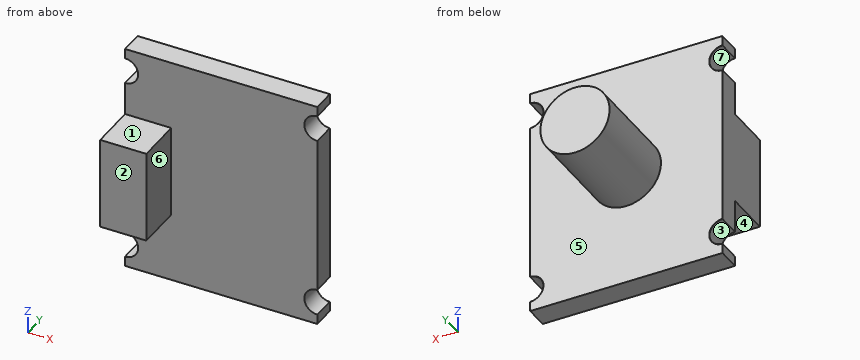
```python
from build123d import *

# Parameters (mm, degrees)
SKETCH1_W                      = 25
SKETCH1_H                      = 30
BOSS_EXTRUDE1_DEPTH            = 3
M3_CLEARANCE_HOLE1_D           = 3.4
M3_CLEARANCE_HOLE1_CSINK_D     = 3.45
M3_CLEARANCE_HOLE1_CSINK_ANGLE = 90
SKETCH4_R                      = 4.5
BOSS_EXTRUDE2_DEPTH            = 12.4
SKETCH5_W                      = 6
SKETCH5_H                      = 12
BOSS_EXTRUDE3_DEPTH            = 6


with BuildPart() as part:
    # Sketch1 → Boss-Extrude1 (new body)
    with BuildSketch(Plane(origin=(0, 0, 0), x_dir=(1, 0, 0), z_dir=(0, 1, 0))):
        with Locations((12.5, 15)):
            Rectangle(SKETCH1_W, SKETCH1_H)
    extrude(amount=BOSS_EXTRUDE1_DEPTH)

    # M3 Clearance Hole1 (through all)
    with Locations(Plane(origin=(0, 3, 0), x_dir=(1, 0, 0), z_dir=(0, 1, 0))):
        with Locations((0, 3), (0, 27), (25, 3), (25, 27)):
            CounterSinkHole(M3_CLEARANCE_HOLE1_D / 2, M3_CLEARANCE_HOLE1_CSINK_D / 2, counter_sink_angle=M3_CLEARANCE_HOLE1_CSINK_ANGLE)

    # Sketch4 → Boss-Extrude2 (add)
    with BuildSketch(Plane(origin=(0, 3, 0), x_dir=(1, 0, 0), z_dir=(0, 1, 0))):
        with Locations(Location((12.5, 15, 0), (0, 0, 90))):
            Circle(SKETCH4_R)
    extrude(amount=BOSS_EXTRUDE2_DEPTH)

    # Sketch5 → Boss-Extrude3 (add)
    with BuildSketch(Plane.XZ):
        with Locations((3, -15)):
            Rectangle(SKETCH5_W, SKETCH5_H)
    extrude(amount=BOSS_EXTRUDE3_DEPTH)


solid = part.part
```
Build history of the part. All positions in model axes, mm. Face numbers are marked on the shaded views. A direction names the side the tool comes from. Round coordinates to 2 decimals unless told otherwise and drop trailing zeros. Write each loop counter-clockwise with the first axis right and the second up, starting at its lowest first coordinate (ties: lowest second). Pieces come first, ordered by that corner, then holes.
1) Band-saw the part on A-A, the plane z = -15. List the corners of the cut face in (x, y), and give its area (3 significant figures).
2) Band-saw the part on D-D, the plane z = -7. List the corners of the cut face in (x, y), and give its area (3 significant figures).
3) 3-axis set-ups, long thin cutter, end or side, ignore diameter. For the marked faces 5, 6 and 7: which of +Z, -Z, +X, -X, +Y, -Y reach the whole face in a straight line?
4) Mould opens along Z. For the marked faces 1, 2, 3 and 4 say: +Z half, -Z half, draft (parallel to the pull), parting line (faces both ways), or undercut.
5) Band-saw the part on C-C, the plane y = 7.5. List the corners of the cut face in (x, z).
6) Pin check, flat tips, straight feed: pin 1 (1.5 mm diameter, centred on x = 10.5, y = 4, fed in from +Z); pin 2 (3 mm diameter, centred on x = 3.5, y = -4, fed in from +Z); pin 3 (3 mm diameter, centred on x = 3, y = -2, fed in from -Z); pin 4 (8 mm diameter, centred on y = 8, z = -5.5, fed in from +X). Stop position of each tip, or through.
7) Drill centre lines: probe 1 along Y at (x, z) = (4.5, -13); probe 2 along Y at (x, z) = (18.75, -6); probe 3 along X at (y, z) = (-0.5, -12.25). Where is each one in solid material? Low to high.
8) Band-saw the part on B-B, the plane x = 12.5. List the corners of the cut face in (y, z), and give its area (3 significant figures).
Ans:
1. outline: (0, -6) - (6, -6) - (6, 0) - (25, 0) - (25, 3) - (17, 3) - (17, 15.4) - (8, 15.4) - (8, 3) - (0, 3) - close
1. area: 223 mm2
2. outline: (0, 0) - (25, 0) - (25, 3) - (0, 3) - close
2. area: 75.0 mm2
3. face 5: +Y
3. face 6: +Z, -Z, +X, -Y
3. face 7: -X, +Y, -Y
4. face 1: +Z half
4. face 2: draft
4. face 3: undercut
4. face 4: -Z half
5. outline: circle Ø9 at (12.5, -15)
6. pin 1: stops at z = -10.68
6. pin 2: stops at z = -9
6. pin 3: stops at z = -21
6. pin 4: passes through
7. probe 1: y = -6 to 3
7. probe 2: y = 0 to 3
7. probe 3: x = 0 to 6
8. outline: (0, -30) - (3, -30) - (3, -19.5) - (15.4, -19.5) - (15.4, -10.5) - (3, -10.5) - (3, 0) - (0, 0) - close
8. area: 202 mm2
